Build history of the part. All positions in model axes, mm. Coordinates: 2 decimals unless noted, no trailing zeros. Order: outer loops, then holes, each group sorted by start corner. A loop starts at its lowest first (then second) coordinate and runs counter-clockwise, first axis right, second up. Notation, with made-up numbers: (37, 29.5) - (62, 29.5) arc R12 cw to (62, 37.5) - close; hole circle Ø8 at (87, 17). An arc over 180 degrees is marked (long way). Return JSON: item names as keys, results as strings.
from build123d import *

# Parameters (mm, degrees)
SKETCH_1_R      = 3.5
SKETCH_1_R_2    = 3.6
SKETCH_1_R_3    = 1.249999971
SKETCH_1_R_4    = 1.75
SKETCH_1_W      = 42.9
SKETCH_1_H      = 33.2
EXTRUDE_1_DEPTH = 2.54


with BuildPart() as part:
    # 草图1 → 凸台-拉伸1 (new body)
    with BuildSketch(Plane(origin=(0, 0, 0), x_dir=(1, 0, 0), z_dir=(0, 1, 0))):
        with BuildLine():
            Line((48.4, -37.799999853), (48.4, -30.444151853))
            add(Edge.make_bspline(
                [(48.4, -30.444151853), (48.4, -30.412185559), (48.381122931, -30.385679038), (48.362542068, -30.359588441), (48.331618599, -30.349282131)],
                knots=[0, 0, 0, 0.5, 0.5, 1, 1, 1], degree=2))
            Line((48.331618599, -30.349282131), (47.2, -29.972075797))
            Line((47.2, -29.972075797), (47.2, -9.827924497))
            Line((47.2, -9.827924497), (48.331621786, -9.450717896))
            add(Edge.make_bspline(
                [(48.331621786, -9.450717896), (48.361949426, -9.440608674), (48.381126465, -9.414316076), (48.400002612, -9.388436014), (48.399998982, -9.35583844)],
                knots=[0, 0, 0, 0.5, 0.5, 1, 1, 1], degree=2))
            Line((48.399998982, -9.35583844), (48.399998982, -2.000000147))
            add(Edge.make_bspline(
                [(48.399998982, -2.000000147), (48.399998982, -1.622352729), (48.255370094, -1.272901625), (48.11105262, -0.924202959), (47.843501866, -0.656497263), (47.576728704, -0.389569608), (47.227097503, -0.244629035), (46.878218161, -0.100000147), (46.499998982, -0.100000147)],
                knots=[0, 0, 0, 0.25, 0.25, 0.5, 0.5, 0.75, 0.75, 1, 1, 1], degree=2))
            Line((46.499998982, -0.100000147), (-46.499999902, -0.100000147))
            add(Edge.make_bspline(
                [(-46.499999902, -0.100000147), (-46.87764732, -0.100000147), (-47.227098424, -0.244629035), (-47.575797089, -0.388946508), (-47.843502786, -0.656497263), (-48.110430441, -0.923270425), (-48.255371014, -1.272901625), (-48.399999902, -1.621780968), (-48.399999902, -2.000000147)],
                knots=[0, 0, 0, 0.25, 0.25, 0.5, 0.5, 0.75, 0.75, 1, 1, 1], degree=2))
            Line((-48.399999902, -2.000000147), (-48.399999902, -9.355848147))
            add(Edge.make_bspline(
                [(-48.399999902, -9.355848147), (-48.399999902, -9.387814441), (-48.381122833, -9.414320961), (-48.362541971, -9.440411559), (-48.331618501, -9.450717869)],
                knots=[0, 0, 0, 0.5, 0.5, 1, 1, 1], degree=2))
            Line((-48.331618501, -9.450717869), (-47.199999902, -9.827924203))
            Line((-47.199999902, -9.827924203), (-47.199999902, -29.97207609))
            Line((-47.199999902, -29.97207609), (-48.331620003, -30.349282599))
            add(Edge.make_bspline(
                [(-48.331620003, -30.349282599), (-48.361947916, -30.359391659), (-48.381125177, -30.385684352), (-48.400001544, -30.411564511), (-48.399997915, -30.444162293)],
                knots=[0, 0, 0, 0.5, 0.5, 1, 1, 1], degree=2))
            Line((-48.399997915, -30.444162293), (-48.4, -37.799999853))
            add(Edge.make_bspline(
                [(-48.4, -37.799999853), (-48.4, -38.177647271), (-48.255371112, -38.527098375), (-48.111053639, -38.875797041), (-47.843502884, -39.143502737), (-47.576729722, -39.410430392), (-47.227098521, -39.555370965), (-46.878219179, -39.699999853), (-46.5, -39.699999853)],
                knots=[0, 0, 0, 0.25, 0.25, 0.5, 0.5, 0.75, 0.75, 1, 1, 1], degree=2))
            Line((-46.5, -39.699999853), (46.5, -39.699999853))
            add(Edge.make_bspline(
                [(46.5, -39.699999853), (46.877647417, -39.699999853), (47.227098521, -39.555370965), (47.575797187, -39.411053492), (47.843502884, -39.143502737), (48.110430539, -38.876729575), (48.255371112, -38.527098375), (48.4, -38.178219032), (48.4, -37.799999853)],
                knots=[0, 0, 0, 0.25, 0.25, 0.5, 0.5, 0.75, 0.75, 1, 1, 1], degree=2))
        make_face()
        with Locations(Location((-34.399999902, -9.900000147, 0), (0, 0, 270))):
            Circle(SKETCH_1_R, mode=Mode.SUBTRACT)
        with Locations(Location((-34.399999902, -29.900000147, 0), (0, 0, 270))):
            Circle(SKETCH_1_R, mode=Mode.SUBTRACT)
        with Locations(Location((33.399998982, -19.9, 0), (0, 0, 270))):
            Circle(SKETCH_1_R_2, mode=Mode.SUBTRACT)
        with Locations(Location((-44.85, -36.15, 0), (0, 0, 270))):
            Circle(SKETCH_1_R_3, mode=Mode.SUBTRACT)
        with Locations(Location((44.85, -36.15, 0), (0, 0, 270))):
            Circle(SKETCH_1_R_3, mode=Mode.SUBTRACT)
        with Locations(Location((27.399998982, -7.899999853, 0), (0, 0, 270))):
            Circle(SKETCH_1_R_4, mode=Mode.SUBTRACT)
        with Locations(Location((-44.85, -3.65, 0), (0, 0, 270))):
            Circle(SKETCH_1_R_3, mode=Mode.SUBTRACT)
        with Locations(Location((44.85, -3.65, 0), (0, 0, 270))):
            Circle(SKETCH_1_R_3, mode=Mode.SUBTRACT)
        with Locations(Location((39.399998982, -7.899999853, 0), (0, 0, 270))):
            Circle(SKETCH_1_R_4, mode=Mode.SUBTRACT)
        with Locations(Location((33.399998982, -31.90000044, 0), (0, 0, 270))):
            Circle(SKETCH_1_R_4, mode=Mode.SUBTRACT)
        with Locations(Location((33.399998982, -7.899999853, 0), (0, 0, 270))):
            Circle(SKETCH_1_R_4, mode=Mode.SUBTRACT)
        with Locations((0, -19.900000147)):
            Rectangle(SKETCH_1_W, SKETCH_1_H, mode=Mode.SUBTRACT)
    extrude(amount=EXTRUDE_1_DEPTH)


solid = part.part
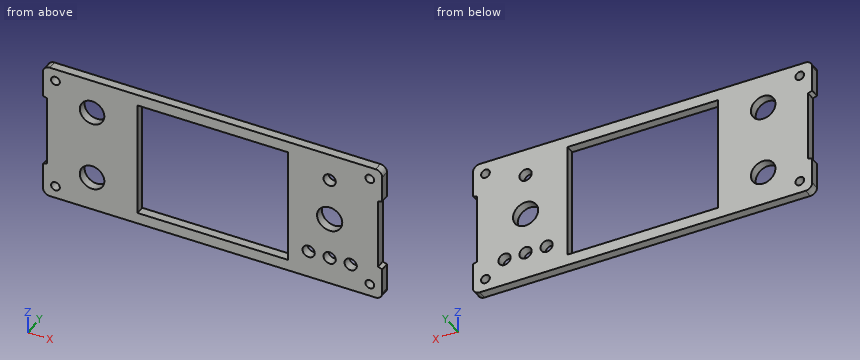
1. Probe L1, parallel to X at y = 0.6, z = 9.9; L2, parallel to X at y = 0.7, z = 36.15; L3, parallel to X at y = 1.4, z = 19.9. List the from-to ranges inside material, lowest first.
Check values:
{"L1": "-47.2 to -37.9, -30.9 to -21.45, 21.45 to 47.2", "L2": "-48.4 to -46.1, -43.6 to -21.45, 21.45 to 43.6, 46.1 to 48.4", "L3": "-47.2 to -21.45, 21.45 to 29.8, 37 to 47.2"}
2. Cut at D-D on z = 31.9. Give the cut face in (x, y).
Check values:
{"outline": "(-48.4, 0) - (-37.27, 0) - (-37.27, 2.54) - (-48.4, 2.54) - close; (-31.53, 0) - (-21.45, 0) - (-21.45, 2.54) - (-31.53, 2.54) - close; (21.45, 0) - (31.65, 0) - (31.65, 2.54) - (21.45, 2.54) - close; (35.15, 0) - (48.4, 0) - (48.4, 2.54) - (35.15, 2.54) - close"}
3. Cut at C-C on x = -34.4. Give the cut face in (y, z).
Check values:
{"outline": "(0, 0.1) - (2.54, 0.1) - (2.54, 6.4) - (0, 6.4) - close; (0, 13.4) - (2.54, 13.4) - (2.54, 26.4) - (0, 26.4) - close; (0, 33.4) - (2.54, 33.4) - (2.54, 39.7) - (0, 39.7) - close"}
4. Drop flat-ended pins along their axis: pin 1 (4 mm diameter, centred on x = -44.85, z = 36.15, fed in from +Y); pin 2 (0.8 mm diameter, centred on y = 1, z = 23, fed in from -X); pin 3 (1 mm diameter, centred on y = 2, z = 15, fed in from +X). Give the stop position or say it passes through.
Check values:
{"pin 1": "y = 2.54", "pin 2": "x = -47.2", "pin 3": "x = 47.2"}
5. Cut at B-B on z = 19.9. Give the cut face in (x, y), plus the area to 3 significant figures.
Check values:
{"outline": "(-47.2, 0) - (-21.45, 0) - (-21.45, 2.54) - (-47.2, 2.54) - close; (21.45, 0) - (29.8, 0) - (29.8, 2.54) - (21.45, 2.54) - close; (37, 0) - (47.2, 0) - (47.2, 2.54) - (37, 2.54) - close", "area": "113 mm²"}
6. Cut at A-A on x = -6. Give the cut face in (y, z), plus the area to 3 significant figures.
Check values:
{"outline": "(0, 0.1) - (2.54, 0.1) - (2.54, 3.3) - (0, 3.3) - close; (0, 36.5) - (2.54, 36.5) - (2.54, 39.7) - (0, 39.7) - close", "area": "16.3 mm²"}
